Autodesk Inventor part; units mm, degrees
ref_plane "YZ Plane" through (0, 0, 0) normal (1, 0, 0) x (0, 1, 0)
ref_plane "XZ Plane" through (0, 0, 0) normal (0, 1, 0) x (-1, 0, 0)
ref_plane "XY Plane" through (0, 0, 0) normal (0, 0, 1) x (1, 0, 0)
sketch "Sketch1" plane through (0, 0, 0) normal (0, 1, 0) x (-1, 0, 0)
  line L0 (-6.35, -3.6662) -> (-6.35, 3.6662)
  line L1 (-6.35, 3.6662) -> (0, 7.3323)
  line L2 (0, 7.3323) -> (6.35, 3.6662)
  line L3 (6.35, 3.6662) -> (6.35, -3.6662)
  line L4 (6.35, -3.6662) -> (0, -7.3323)
  line L5 (0, -7.3323) -> (-6.35, -3.6662)
  circle A0 centre (0, 0) radius 6.35
  circle A1 centre (0, 0) radius 9.35
  dimension "d0" = 12.7
  dimension "d1" = 3
extrude "Extrusion1" add sketch "Sketch1" along normal blind 3 contours L0 A0 L5 | L0 L1 A0 | A0 | A0 L4 L5 | L1 L2 A0 | A0 L3 L4 | L2 L3 A0 | A1
sketch "Sketch2" plane through (0, 3, 0) normal (0, 1, 0) x (1, 0, 0)
  line L0 (-7.347, 0) -> (-3.6735, 6.3627)
  line L1 (-3.6735, 6.3627) -> (3.6735, 6.3627)
  line L2 (3.6735, 6.3627) -> (7.347, 0)
  line L3 (7.347, 0) -> (3.6735, -6.3627)
  line L4 (3.6735, -6.3627) -> (-3.6735, -6.3627)
  line L5 (-3.6735, -6.3627) -> (-7.347, 0)
  point P0 (0, 0)
  point P1 (0, 0)
  dimension "d4" = 12.7254
extrude "Extrusion2" cut sketch "Sketch2" against normal blind 3
properties part number "3mmHEXSPACER"
Input: part model. Units: mm. Frame: model coordinates. A direction names the side the tool comes from. Round coordinates to 2 decimals unless told otherwise and drop trailing zeros. Loops run counter-clockwise (first coordinate to the right, second up) from the corner with the lowest first, then second, coordinate; pieces in that order, holes last. Notation, with made-up numbers: (32, 4) -> (81, 4) arc R27 cw to (81, 25) -> close; hole circle Ø5 at (57.25, 44). An arc over 180 degrees is marked (long way). Write each question's results on one line, items separated by ' | '.
1. Section A-A (x = 0). Return loops of the section in (y, z).
Geometry results:
outline: (0, -9.35) -> (3, -9.35) -> (3, -6.36) -> (0, -6.36) -> close; (0, 6.36) -> (3, 6.36) -> (3, 9.35) -> (0, 9.35) -> close
2. First-contact query: P1, Ø1.5, axis at y = 1, z = 7, coming from the +X side; P2, Ø1.5, axis at x = -5, y = 1, coming from the +Z side. Flat tips, straight axial feed; report the tip coordinate or a pass-through.
Geometry results:
P1: x = 6.95 | P2: z = 8.33
3. Section C-C (z = -0.75). Return loops of the section in (x, y).
Geometry results:
outline: (-9.32, 0) -> (-6.91, 0) -> (-6.91, 3) -> (-9.32, 3) -> close; (6.91, 0) -> (9.32, 0) -> (9.32, 3) -> (6.91, 3) -> close
4. Section D-D (z = -7.5). Return loops of the section in (x, y).
Geometry results:
outline: (-5.58, 0) -> (5.58, 0) -> (5.58, 3) -> (-5.58, 3) -> close
5. Section B-B (y = 0.45). Return loops of the section in (x, z), and give its area (3 significant figures).
Geometry results:
outline: circle Ø18.7 at (0, 0); hole (-7.35, 0) -> (-3.67, -6.36) -> (3.67, -6.36) -> (7.35, 0) -> (3.67, 6.36) -> (-3.67, 6.36) -> close | area: 134 mm2
6. Set-up query: faces 1 (the face through (6.4, 3, 2.2)), 2 (the face through (-5.5, 1.5, 3.2)). Return all of +Z, -Z, +X, -X, +Y, -Y with unobstructed straight access to the full face (end or side cutting, diameter ignored); none if empty.
Geometry results:
face 1: +Z, -Z, +X, -X, +Y | face 2: +Y, -Y
7. Ray query, line 1 (Z direction, x = 6, y = 1.2); line 2 (X direction, y = 0.2, z = -3.5); line 3 (X direction, y = 2.55, z = 2). Return the intervals inside material, ascending. Write a range as from..to.
Geometry results:
line 1: -7.17..-2.33, 2.33..7.17 | line 2: -8.67..-5.33, 5.33..8.67 | line 3: -9.13..-6.19, 6.19..9.13
8. Mould query, pull axis X, two halves, no side actions, for faces 3 (the face through (-5.536, 1.521, -3.137)), 4 (the face through (2.027, 1.479, 9.128)), 5 (the face through (6.4, 0, 2.2)). Classes: +X half, -X half, draft (parallel to the pull), parting line (faces both ways), or undercut.
Geometry results:
face 3: undercut | face 4: parting line | face 5: draft
